Source: CAD feature listing. Evaluate the final solid. Frame: model axes, mm. A direction names the side the tool comes from. Coordinates: 2 decimals unless noted, no trailing zeros. Loops run counter-clockwise (first coordinate to the right, second up) from the corner with the lowest first, then second, coordinate; pieces in that order, holes last. Notation, with made-up numbers: M 12.5,-15 L 43.5,-15 A29 ccw 43.5,18 Z; hole C -31,-31 d7. An arc over 180 degrees is marked long. Write each question's results on one line, items separated by ' | '. Start each with the question number.
from build123d import *

# Parameters (mm, degrees)
F0_W     = 5
F0_H     = 15
F1_DEPTH = 12
F2_W     = 5
F2_H     = 5
F3_DEPTH = 5
F4_R     = 2.49999
F6_D     = 3.3


# Not quite as in the source:
# - a fillet or chamfer is up to 0.001 mm smaller than in the source, because OpenCascade refuses the exact size


with BuildPart() as f1:
    # F0 (on Top) → F1 (new body)
    with BuildSketch(Plane.XY):
        Rectangle(F0_W, F0_H)
    extrude(amount=F1_DEPTH)

    # F2 (on face) → F3 (cut, through all)
    with BuildSketch(Plane.YZ.offset(2.5)):
        with Locations((0, 6)):
            Rectangle(F2_W, F2_H)
    extrude(amount=-F3_DEPTH, mode=Mode.SUBTRACT)

    # F4 (radius 2.5 in the source; OpenCascade refuses exactly that, so slightly less here)
    f4_edges = [f1.edges().sort_by_distance(p)[0] for p in [
        (2.5, -7.5, 6),
        (-2.5, -7.5, 6),
        (2.5, 7.5, 6),
        (-2.5, 7.5, 6),
        (-2.5, 2.5, 6),
        (-2.5, -2.5, 6),
        (2.5, -2.5, 6),
        (2.5, 2.5, 6),
    ]]
    fillet(f4_edges, radius=F4_R)

    # F6 (through all)
    with Locations(Plane.XY.offset(12)):
        with Locations((0, 5), (0, -5)):
            Hole(F6_D / 2)


solid = f1.part
Item 1: Line query: probe 1 along Y at (x, z) = (0, 5.5); probe 2 along Y at (x, z) = (-0.85, 4); probe 3 along Y at (x, z) = (0.1, 11.75). Output: solid intervals per line, ascending.
Item 2: Cut plane B-B (y = 2.25). Output: boundary loops of the cut face in (x, z).
Item 3: Cut plane C-C (x = 0.9). Output: boundary loops of the cut face in (y, z), then the cut area to 3 significant figures.
Item 4: Access query for faces 4 (the cylindrical face through (1.748, 3.213, 6.035)), 5 (the cylindrical face through (1.748, 6.787, 6.084)), 6 (the cylindrical face through (-1.787, -3.252, 6.035)). Directions: +Z, -Z, +X, -X, +Y, -Y. A direction counts if a zero-diameter tool reaches every point of the face in a straight line with its end or side. Return the directions, or none.
Item 5: First-contact query: pin 1 Ø1.5 at (x, z) = (-1.5, 3.5) entering from +Y. Flat tip, straight axial feed; report the tip coordinate or a pass-through.
Item 6: Cut plane A-A (z = 4). Count the separate pieces of the cut face and the enclosed holes in it, then the cut area to 3 significant figures.
Item 7: Mould query, pull axis Y, two halves, no side actions, for faces 1 (the flat face through (0, 0, 12)), 2 (the cylindrical face through (1.748, -3.213, 6.035)), 3 (the cylindrical face through (-1.787, -6.748, 6.084)). Classes: +Y half, -Y half, draft (parallel to the pull), parting line (faces both ways), or undercut.
Response values:
1) probe 1: y = -7.5 to -6.65, -3.35 to -2.5, 2.5 to 3.35, 6.65 to 7.5 | probe 2: y = -7.35 to -6.41, -3.59 to -2.65, 2.65 to 3.59, 6.41 to 7.35 | probe 3: y = -7.5 to -6.65, -3.35 to 3.35, 6.65 to 7.5
2) outline: M -2.5,0 L 2.5,0 L 2.5,3.5 L -2.5,3.5 Z; M -2.5,8.5 L 2.5,8.5 L 2.5,12 L -2.5,12 Z
3) outline: M -7.33,0 L -6.38,0 L -6.38,12 L -7.33,12 Z; M -3.62,0 L 3.62,0 L 3.62,12 L -3.62,12 Z; M 6.38,0 L 7.33,0 L 7.33,12 L 6.38,12 Z; hole M -2.67,3.5 L 2.67,3.5 L 2.67,8.5 L -2.67,8.5 Z | area: 82.9 mm2
4) face 4: +X | face 5: +Z, -Z, +X, +Y | face 6: -X
5) pin 1: stops at y = 7.38
6) separate pieces: 2 | enclosed holes: 2 | area: 22.2 mm2
7) face 1: draft | face 2: undercut | face 3: -Y half
